CAD build for the part. Positions are in the model's coordinates, mm. A direction names the side the tool comes from. Coordinates: 2 decimals unless noted, no trailing zeros. Loops run counter-clockwise (first coordinate to the right, second up) from the corner with the lowest first, then second, coordinate; pieces in that order, holes last.
1) Pin check, flat tips, straight feed: pin 1 Ø1.2 at (y, z) = (-7.5, 0) entering from +X; pin 2 Ø2 at (x, y) = (4.5, 2.5) entering from -Z; pin 3 Ø2 at (y, z) = (5.5, -1) entering from +X (3 decimals). Stop position of each tip, or through.
2) Which spindle directions (+Z, -Z, +X, -X, +Y, -Y) get a long thin tool onto all of the face, cutting with end or side? Do faces 1 (the cylindrical face through (0.258, -6.605, -0.034)), 2 (the flat face through (21.412, 0, 0)), 3 (the flat face through (0.508, -7, 0)), 4 (the flat face through (-11.608, 0, 0)). Say none if no direction does.
3) Saw through at D-D, the plane y = -9.25. Write the cut outline in (x, z), and give its area (3 significant figures).
4) Two-plate mould, pull along Y, no slides. Class faces 5 (the cylindrical face through (-5.9, 8.2, -7.5)), 6 (the flat face through (22.225, 1, 0)), 7 (the flat face through (22, -0.406, 0)): +Y half, -Y half, draft (parallel to the pull), parting line (faces both ways), or undercut.
5) Wall check: line 1 along X through (y, z) = (-6.5, 6.5); line 2 along Z through (x, y) = (-2, 0); line 3 along X through (y, z) = (-2.25, 4) (3 decimals). Give the ranges that are in metal, low to high.
6) Saw through at C-C, the plane x = 6. Write the cut outline in (y, z) (1 decimal).
```python
from build123d import *

# Parameters (mm, degrees)
SKETCH3_R               = 0.762
BOSS_EXTRUDE1_DEPTH     = 0.508
CUT_EXTRUDE1_DEPTH      = 28.219954767
CUT_EXTRUDE1_DEPTH_BACK = 28.219954767
SKETCH4_W               = 0.8128
SKETCH4_H               = 0.8128
CHAMFER1_SIZE           = 0.4064


with BuildPart() as part:
    # Sketch2 → Revolve1 (revolve)
    with BuildSketch(Plane.XY, mode=Mode.PRIVATE) as revolve1_sk:
        Polygon((0, 0), (22.225, 0), (22.225, 3.17119), (9.525, 3.17119), (9.525, 4.7625), (1.4986, 4.7625), (1.4986, 5.1562), (0, 5.1562), (0, 11.1125), (-11.6078, 11.1125), (-11.6078, 0), align=None)
    revolve(revolve1_sk.sketch.rotate(Axis((22.225, 0, 0), (1, 0, 0)), 180), axis=Axis((22.225, 0, 0), (1, 0, 0)))

    # Sketch3 → Boss-Extrude1 (add, symmetric)
    with BuildSketch(Plane(origin=(0, 0, 0), x_dir=(0, 0, -1), z_dir=(1, 0, 0))):
        with Locations(Location((0, -7.366, 0), (0, 0, 270))):
            Circle(SKETCH3_R)
    extrude(amount=BOSS_EXTRUDE1_DEPTH, both=True)

    # Sketch4 → Cut-Extrude1 (cut, two sides: drawn at the far end of the back side and taken through both)
    with BuildSketch(Plane.XY.offset(-CUT_EXTRUDE1_DEPTH_BACK)):
        with Locations((21.8186, 0)):
            Rectangle(SKETCH4_W, SKETCH4_H)
    extrude(amount=CUT_EXTRUDE1_DEPTH + CUT_EXTRUDE1_DEPTH_BACK, mode=Mode.SUBTRACT)

    # Chamfer1
    chamfer1_edges = [part.edges().sort_by_distance(p)[0] for p in [
        (22.225, 3.17119, 0),
        (22.225, -2.381723917, 2.093761496),
    ]]
    chamfer(chamfer1_edges, length=CHAMFER1_SIZE)


solid = part.part
```
Data:
1. pin 1: stops at x = 0.51
1. pin 2: stops at z = -4.52
1. pin 3: stops at x = 9.525
2. face 1: +X
2. face 2: +Z, -Z, +X
2. face 3: +Z, -Z, +X, -Y
2. face 4: +Z, -Z, -X, +Y, -Y
3. outline: (-11.61, -6.16) - (0, -6.16) - (0, 6.16) - (-11.61, 6.16) - close
3. area: 143 mm2
4. face 5: parting line
4. face 6: draft
4. face 7: undercut
5. line 1: x = -11.61 to 0
5. line 2: z = -11.11 to 11.11
5. line 3: x = -11.608 to 9.525
6. outline: circle Ø9.5 at (0, 0)
